```python
from build123d import *

# Parameters (mm, degrees)
CHAMFER1_SIZE  = 1
CHAMFER1_SIZE2 = 0.267949192
CHAMFER2_SIZE  = 1.5


with BuildPart() as part:
    # Sketch1 → Revolve1 (revolve)
    with BuildSketch(Plane(origin=(0, 0, 0), x_dir=(1, 0, 0), z_dir=(0, 1, 0))):
        Polygon((0, 0), (12.5, 0), (12.5, 3), (10, 3), (10, 9), (7.5, 9), (7.5, 18.2), (7.15, 18.2), (7.15, 19.8), (7.5, 19.8), (7.5, 21), (0, 21), align=None)
    revolve(axis=Axis((0, 0, 0), (0, 0, -1)))

    # Chamfer1
    chamfer1_edges = [part.edges().sort_by_distance(p)[0] for p in [
        (-7.5, 0, -21),
    ]]
    chamfer1_side = [part.faces().sort_by_distance(p)[0] for p in [
        (0, 0, -21),
    ]]
    chamfer(chamfer1_edges, length=CHAMFER1_SIZE, length2=CHAMFER1_SIZE2, reference=chamfer1_side[0])

    # Chamfer2
    chamfer2_edges = [part.edges().sort_by_distance(p)[0] for p in [
        (-10, 0, -9),
    ]]
    chamfer(chamfer2_edges, length=CHAMFER2_SIZE)


solid = part.part
```
Source: CAD feature listing. Evaluate the final solid. Frame: model axes, mm. A direction names the side the tool comes from. Round coordinates to 2 decimals unless told otherwise and drop trailing zeros. Loops run counter-clockwise (first coordinate to the right, second up) from the corner with the lowest first, then second, coordinate; pieces in that order, holes last.
1. Section query A-A on x = 0. Output: boundary loops of the cut face in (y, z).
2. Access query for faces 1 (the flat face through (0, 0, -21)), 2 (the cylindrical face through (-0.93, -7.09, -19.01)), 3 (the flat face through (0, 8, -9)). Directions: +Z, -Z, +X, -X, +Y, -Y. A direction counts if a zero-diameter tool reaches every point of the face in a straight line with its end or side. Return the directions, or none.
3. Ray query, L1, parallel to Z at x = -7.5, y = 3.25; L2, parallel to Z at x = 6.5, y = -0.5; L3, parallel to Y at x = 0.25, z = -6.25. Return the intervals inside material, ascending.
4. Section query D-D on z = -6. Output: boundary loops of the cut face in (x, y).
5. Section query C-C on z = -18.75. Output: boundary loops of the cut face in (x, y).
6. Contact query for flat-ended pins moving along their axis: pin 1 (5 mm diameter, centred on x = 1.5, y = -7.5, fed in from -Z); pin 2 (2 mm diameter, centred on x = -6.5, y = -6, fed in from -Z); pin 3 (1.5 mm diameter, centred on x = -4, z = -10, fed in from +Y); pin 4 (6 mm diameter, centred on x = 2, z = -16.5, fed in from +Y). Output: stop coordinate, or through.
Answers below:
1. outline: (-12.5, -3) - (-10, -3) - (-10, -7.5) - (-8.5, -9) - (-7.5, -9) - (-7.5, -18.2) - (-7.15, -18.2) - (-7.15, -19.8) - (-7.5, -19.8) - (-7.5, -20.73) - (-6.5, -21) - (6.5, -21) - (7.5, -20.73) - (7.5, -19.8) - (7.15, -19.8) - (7.15, -18.2) - (7.5, -18.2) - (7.5, -9) - (8.5, -9) - (10, -7.5) - (10, -3) - (12.5, -3) - (12.5, 0) - (-12.5, 0) - close
2. face 1: -Z, +X, -X, +Y, -Y
2. face 2: none
2. face 3: -Z
3. L1: z = -9 to 0
3. L2: z = -20.99 to 0
3. L3: y = -10 to 10
4. outline: circle Ø20 at (0, 0)
5. outline: circle Ø14.3 at (0, 0)
6. pin 1: stops at z = -21
6. pin 2: stops at z = -9
6. pin 3: stops at y = 6.76
6. pin 4: stops at y = 7.5
